Design review of the part built by this model. Coordinates are the model's own, in mm. Face numbers are marked on the shaded views. A direction names the side the tool comes from. Round coordinates to 2 decimals unless told otherwise and drop trailing zeros. Order: outer loops, then holes, each group sorted by start corner. A loop starts at its lowest first (then second) coordinate and runs counter-clockwise, first axis right, second up. Notation, with made-up numbers: M 38.25,-32 L 79.25,-32 A29 ccw 79.25,6 Z; hole C -36,45 d6. An arc over 180 degrees is marked long. Use a Markdown table: item, result. Add a question column.
(1) Take a section at D-D (y = 12). Write out the cut boundary in (x, z), then the cut area to 3 significant figures.
(2) Machinability: for the marked faces 1 and 2, which of the approach directions +Z, -Z, +X, -X, +Y, -Y give a long, thin tool a straight path to every point of the face, cutting with its end or side? Answer none if there is none.
(3) The part is to be moulded in two halves that separate along Y. For the marked faces 3, 4 and 5, say which applies: released by +Y, released by -Y, zero draft, split by the parting line, or undercut.
(4) For pin 1 (9 mm diameter, centred on y = 10.5, z = 26.5, fed in from +X); pin 2 (1.5 mm diameter, centred on x = -24.5, z = 17, fed in from -Y); pin 3 (1.5 mm diameter, centred on y = 8, z = 6, fed in from +X); pin 4 (11.5 mm diameter, centred on x = -6.5, y = 21.5, fed in from +Z), all flat-tipped, find the tip position at first contact; note any pin that passes through.
(5) Take a section at B-B (x = -12). Write out the cut boundary in (y, z).
(6) Take a section at C-C (z = 33). Write out the cut boundary in (x, y).
(7) Take a section at A-A (y = 15). Write out the cut boundary in (x, z).
(8) To check wall thickness, follow probe 1 along Y at (x, z) = (-12, 3.15); probe 2 along Y at (x, z) = (-26, 34); probe 3 along Z at (x, y) = (-25.6, 5). State the ranges of each line that lie inside material, in increasing order. Write a range as from..to.
```python
from build123d import *

# Parameters (mm, degrees)
F0_W     = 25
F0_H     = 30
F0_R     = 9.25
F0_W_2   = 3
F1_DEPTH = 5
F2_DEPTH = 40
F3_R     = 10
F4_R     = 1.75
F5_DEPTH = 3.001
F6_R     = 2


with BuildPart() as f1:
    # F0 (on Top) → F1 (new body)
    with BuildSketch(Plane.XY):
        with Locations((-12.5, 15)):
            Rectangle(F0_W, F0_H)
        with Locations((-12, 15)):
            Circle(F0_R, mode=Mode.SUBTRACT)
        with Locations((-26.5, 15)):
            Rectangle(F0_W_2, F0_H)
    extrude(amount=F1_DEPTH)

    # F0 (on Top) → F2 (join)
    with BuildSketch(Plane.XY):
        with Locations((-26.5, 15)):
            Rectangle(F0_W_2, F0_H)
    extrude(amount=F2_DEPTH)

    # F3
    f3_edges = [f1.edges().sort_by_distance(p)[0] for p in [
        (0, 0, 2.5),
        (0, 30, 2.5),
    ]]
    fillet(f3_edges, radius=F3_R)

    # F4 (on face) → F5 (cut, through all)
    with BuildSketch(Plane.YZ.offset(-25)):
        with Locations((5, 32.5)):
            Circle(F4_R)
        with BuildLine():
            ThreePointArc((25.8762976423, 34.0147945214), (26.5159190074, 33.3743509381), (26.75, 32.5))
            ThreePointArc((26.75, 32.5), (26.5151696279, 31.6243510986), (25.8737017159, 30.9837067198))
            ThreePointArc((25.8737017159, 30.9837067198), (26.2572446424, 30.8193071518), (26.6688053839, 30.7503858164))
            Line((26.6688053839, 30.7503858164), (26.8316769531, 30.7504083459))
            ThreePointArc((26.8316769531, 30.7504083459), (28.015984309, 31.290286813), (28.4999993582, 32.4985012412))
            ThreePointArc((28.4999993582, 32.4985012412), (27.9856735638, 33.7376982625), (26.7450173494, 34.2484941496))
            ThreePointArc((26.7450173494, 34.2484941496), (26.2953839701, 34.1884198336), (25.8762976423, 34.0147945214))
        make_face()
        with BuildLine():
            ThreePointArc((25.313264961, 33.4976480132), (25.5661966357, 33.7873422376), (25.8762976423, 34.0147945214))
            ThreePointArc((25.8762976423, 34.0147945214), (25.5235901108, 34.1698363381), (25.1455039627, 34.2439405371))
            Line((25.1455039627, 34.2439405371), (24.8445689194, 34.243083813))
            ThreePointArc((24.8445689194, 34.243083813), (24.6385972754, 34.2122756994), (24.4377440921, 34.1572170329))
            ThreePointArc((24.4377440921, 34.1572170329), (24.9284794863, 33.8977522036), (25.313264961, 33.4976480132))
        make_face()
        with BuildLine():
            ThreePointArc((25.1455039627, 34.2439405371), (25.5235901108, 34.1698363381), (25.8762976423, 34.0147945214))
            ThreePointArc((25.8762976423, 34.0147945214), (26.2953839701, 34.1884198336), (26.7450173494, 34.2484941496))
            Line((26.7450173494, 34.2484941496), (25.1455039627, 34.2439405371))
        make_face()
        with BuildLine():
            ThreePointArc((26.6688053839, 30.7503858164), (26.2572446424, 30.8193071518), (25.8737017159, 30.9837067198))
            ThreePointArc((25.8737017159, 30.9837067198), (25.4635661352, 30.8125147591), (25.0235325622, 30.7501582304))
            Line((25.0235325622, 30.7501582304), (26.6688053839, 30.7503858164))
        make_face()
        with BuildLine():
            ThreePointArc((25.0235325622, 30.7501582304), (25.4635661352, 30.8125147591), (25.8737017159, 30.9837067198))
            ThreePointArc((25.8737017159, 30.9837067198), (25.5644222061, 31.2112923163), (25.3122242271, 31.5008526697))
            ThreePointArc((25.3122242271, 31.5008526697), (24.927751526, 31.1016985717), (24.4377457378, 30.8427824088))
            ThreePointArc((24.4377457378, 30.8427824088), (24.7037063498, 30.7752652167), (24.97695154, 30.750151787))
            Line((24.97695154, 30.750151787), (25.0235325622, 30.7501582304))
        make_face()
        with BuildLine():
            Line((24.8445689194, 34.243083813), (25.1455039627, 34.2439405371))
            ThreePointArc((25.1455039627, 34.2439405371), (24.9950179912, 34.2499929084), (24.8445689194, 34.243083813))
        make_face()
        with BuildLine():
            ThreePointArc((24.97695154, 30.750151787), (25.0002420726, 30.7500000167), (25.0235325622, 30.7501582304))
            Line((25.0235325622, 30.7501582304), (24.97695154, 30.750151787))
        make_face()
        with BuildLine():
            Line((26.8316769531, 30.7504083459), (26.6688053839, 30.7503858164))
            ThreePointArc((26.6688053839, 30.7503858164), (26.7502414308, 30.7485012579), (26.8316769531, 30.7504083459))
        make_face()
        with BuildLine():
            ThreePointArc((24.4377440921, 34.1572170329), (24.6385972754, 34.2122756994), (24.8445689194, 34.243083813))
            Line((24.8445689194, 34.243083813), (24.0543595868, 34.2408341869))
            ThreePointArc((24.0543595868, 34.2408341869), (24.248402903, 34.2098052318), (24.4377440921, 34.1572170329))
        make_face()
        with BuildLine():
            ThreePointArc((24.4377457378, 30.8427824088), (23.25, 32.4999991311), (24.4377440921, 34.1572170329))
            ThreePointArc((24.4377440921, 34.1572170329), (24.248402903, 34.2098052318), (24.0543595868, 34.2408341869))
            Line((24.0543595868, 34.2408341869), (23.6867111794, 34.2397875383))
            ThreePointArc((23.6867111794, 34.2397875383), (22.1280512127, 32.4053512558), (23.8757319025, 30.7499994584))
            ThreePointArc((23.8757319025, 30.7499994584), (24.1605392352, 30.7733706928), (24.4377457378, 30.8427824088))
        make_face()
        with BuildLine():
            Line((23.8757319025, 30.7499994584), (24.97695154, 30.750151787))
            ThreePointArc((24.97695154, 30.750151787), (24.7037063498, 30.7752652167), (24.4377457378, 30.8427824088))
            ThreePointArc((24.4377457378, 30.8427824088), (24.1605392352, 30.7733706928), (23.8757319025, 30.7499994584))
        make_face()
        with BuildLine():
            Line((23.6867111794, 34.2397875383), (24.0543595868, 34.2408341869))
            ThreePointArc((24.0543595868, 34.2408341869), (23.8705078211, 34.2499923501), (23.6867111794, 34.2397875383))
        make_face()
        with BuildLine():
            ThreePointArc((25.8737017159, 30.9837067198), (26.5151696279, 31.6243510986), (26.75, 32.5))
            ThreePointArc((26.75, 32.5), (26.5159190074, 33.3743509381), (25.8762976423, 34.0147945214))
            ThreePointArc((25.8762976423, 34.0147945214), (25.5661966357, 33.7873422376), (25.313264961, 33.4976480132))
            ThreePointArc((25.313264961, 33.4976480132), (25.545610556, 33.0226817163), (25.6254898299, 32.4999994417))
            ThreePointArc((25.6254898299, 32.4999994417), (25.5453379061, 31.9764467676), (25.3122242271, 31.5008526697))
            ThreePointArc((25.3122242271, 31.5008526697), (25.5644222061, 31.2112923163), (25.8737017159, 30.9837067198))
        make_face()
        with BuildLine():
            ThreePointArc((25.3122242271, 31.5008526697), (24.9999995959, 32.4994133448), (25.313264961, 33.4976480132))
            ThreePointArc((25.313264961, 33.4976480132), (24.9284794863, 33.8977522036), (24.4377440921, 34.1572170329))
            ThreePointArc((24.4377440921, 34.1572170329), (23.25, 32.4999991311), (24.4377457378, 30.8427824088))
            ThreePointArc((24.4377457378, 30.8427824088), (24.927751526, 31.1016985717), (25.3122242271, 31.5008526697))
        make_face()
        with BuildLine():
            ThreePointArc((25.6254898299, 32.4999994417), (25.545610556, 33.0226817163), (25.313264961, 33.4976480132))
            ThreePointArc((25.313264961, 33.4976480132), (24.9999995959, 32.4994133448), (25.3122242271, 31.5008526697))
            ThreePointArc((25.3122242271, 31.5008526697), (25.5453379061, 31.9764467676), (25.6254898299, 32.4999994417))
        make_face()
    extrude(amount=-F5_DEPTH, mode=Mode.SUBTRACT)

    # F6
    f6_edges = [f1.edges().sort_by_distance(p)[0] for p in [
        (-25, 15, 5),
    ]]
    fillet(f6_edges, radius=F6_R)


solid = f1.part
```
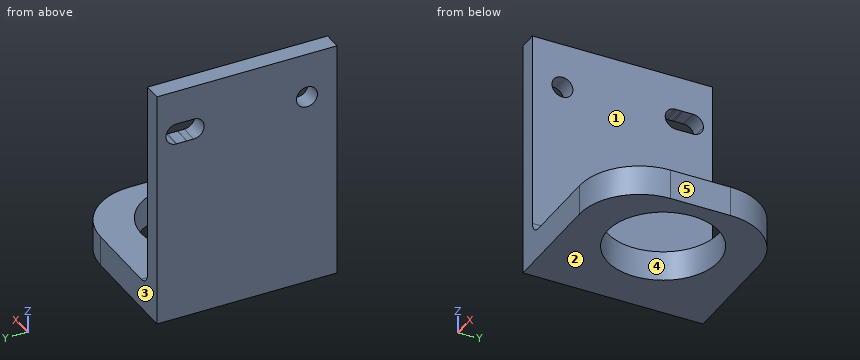
Verdict:
| question | item | result |
|---|---|---|
| 1 | outline | M -28,0 L -20.75,0 L -20.75,5 L -23,5 A2 cw -25,7 L -25,40 L -28,40 Z; M -3.25,0 L 0,0 L 0,5 L -3.25,5 Z |
| 1 | area | 158 mm^2 |
| 2 | face 1 | +Z, +X, +Y, -Y |
| 2 | face 2 | -Z, +X, -X, +Y, -Y |
| 3 | face 3 | released by +Y |
| 3 | face 4 | undercut |
| 3 | face 5 | zero draft |
| 4 | pin 1 | stops at x = -25 |
| 4 | pin 2 | stops at y = 0 |
| 4 | pin 3 | stops at x = -23.97 |
| 4 | pin 4 | stops at z = 5 |
| 5 | outline | M 0,0 L 5.75,0 L 5.75,5 L 0,5 Z; M 24.25,0 L 30,0 L 30,5 L 24.25,5 Z |
| 6 | outline | M -28,0 L -25,0 L -25,3.32 L -28,3.32 Z; M -28,6.68 L -25,6.68 L -25,22.2 L -28,22.2 Z; M -28,28.43 L -25,28.43 L -25,30 L -28,30 Z |
| 7 | outline | M -28,0 L -21.25,0 L -21.25,5 L -23,5 A2 cw -25,7 L -25,40 L -28,40 Z; M -2.75,0 L 0,0 L 0,5 L -2.75,5 Z |
| 8 | probe 1 | y = 0..5.75, 24.25..30 |
| 8 | probe 2 | y = 0..4.1, 5.9..22.97, 27.65..30 |
| 8 | probe 3 | z = 0..30.75, 34.25..40 |
